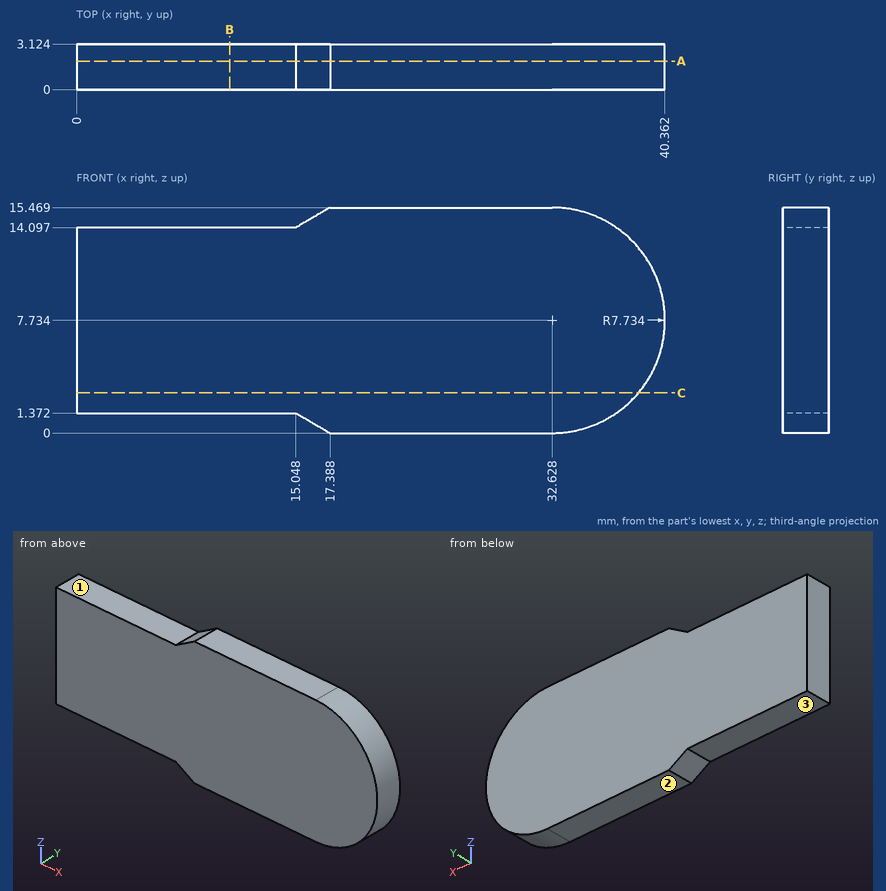
Geometry: see drawing. Coordinates: mm, zero at the bounding-box minimum. A direction names the side the tool comes from. Coordinates: 2 decimals unless noted, no trailing zeros. Write each loop counter-clockwise with the first axis right and the second up, starting at its lowest first coordinate (ties: lowest second). Pieces come first, ordered by that corner, then holes. Notation, with made-up numbers: M 34,20 L 74,20 A27 ccw 74,53 Z; hole C 55.5,22 d1. An arc over 180 degrees is marked long. Use CSV: the item, a comma, the result in double quotes. Start each with the question number.
1. First-contact query: P1, Ø0.9, axis at x = 5.5, y = 2, coming from the -Z side; P2, Ø1, axis at y = 2.5, z = 9.5, coming from the +X side. Flat tips, straight axial feed; report the tip coordinate or a pass-through.
2. Reachability of the marked faces 1, 2 and 3 from +Z, -Z, +X, -X, +Y, -Y: full face, straight path, thin tool, end or side. Return the list, or none.
3. Cut plane C-C on z = 2.75. Return the cut outline in (x, y) (1 decimal).
4. Ray query, probe 1 along Z at (x, y) = (15, 2); probe 2 along Z at (x, y) = (36.5, 0.3); probe 3 along X at (y, z) = (1.65, 14.25) (1 decimal). Return the intervals inside material, ascending.
5. Cut plane A-A on y = 1.95. Return the cut outline in (x, z) (1 decimal).
6. Cut plane B-B on x = 10.5. Return the cut outline in (y, z) (1 decimal).
Entries:
1,P1,"z = 1.37"
1,P2,"x = 40.26"
2,face 1,"+Z, -X, +Y, -Y"
2,face 2,"-Z, +X, -X, +Y, -Y"
2,face 3,"-Z, -X, +Y, -Y"
3,outline,"M 0,0 L 38.5,0 L 38.5,3.1 L 0,3.1 Z"
4,probe 1,"1.37 to 14.1"
4,probe 2,"1.04 to 14.43"
4,probe 3,"15.3 to 36.8"
5,outline,"M 0,1.4 L 15,1.4 L 17.4,0 L 32.6,0 A7.7 ccw 32.6,15.5 L 17.4,15.5 L 15,14.1 L 0,14.1 Z"
6,outline,"M 0,1.4 L 3.1,1.4 L 3.1,14.1 L 0,14.1 Z"
